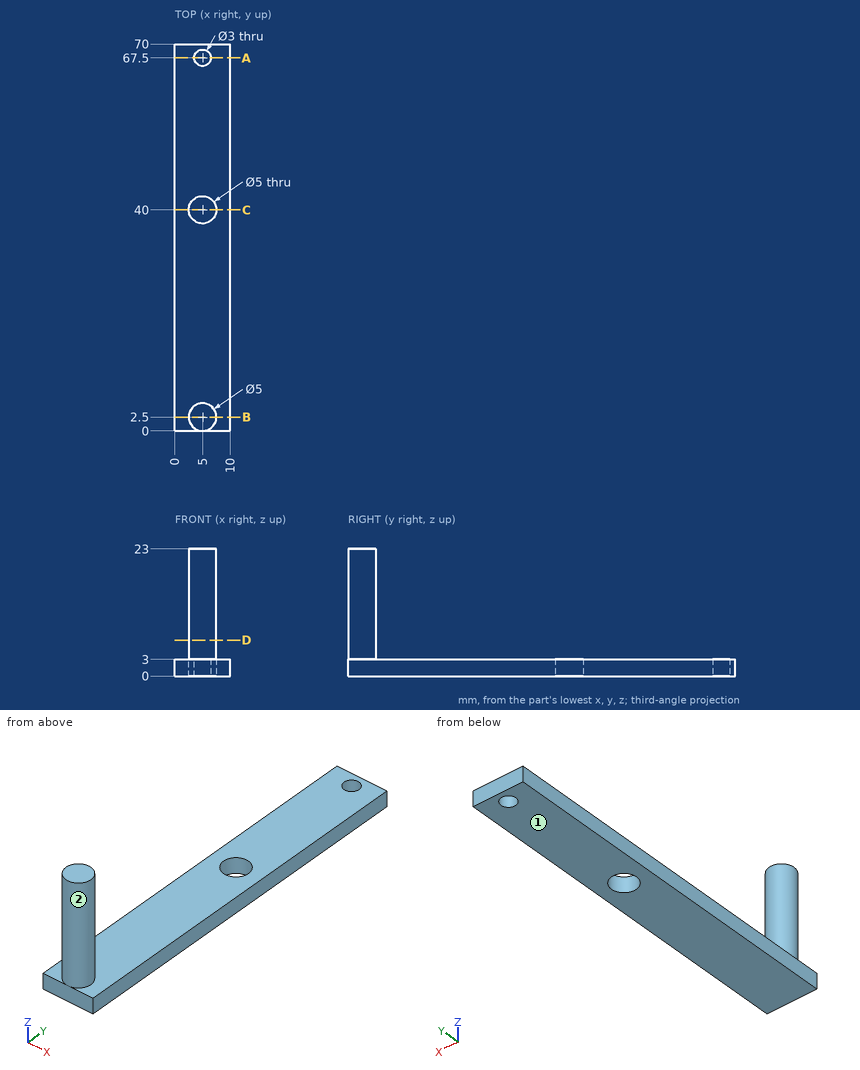
Answer from the drawing. Dimensions are ordinates in mm from the lowest x, y and z of the part. A direction names the side the tool comes from. Coordinates: 2 decimals unless noted, no trailing zeros. Order: outer loops, then holes, each group sorted by start corner. A loop starts at its lowest first (then second) coordinate and runs counter-clockwise, first axis right, second up. Notation, with made-up numbers: M -32.75,25.5 L -26.75,25.5 A33 cw -26.75,60.5 Z; hole C -21.75,15 d11. An arc over 180 degrees is marked long. Put each result on its own line as item: value. Start each with the question number.
Item 1: Section A-A, the plane y = 67.5 is taken. Determine the outline of the cut face in (x, z), plus the area to 3 significant figures.
Item 2: Section D-D, the plane z = 6.5 is taken. Determine the outline of the cut face in (x, y).
Item 3: Consider probe 1 along Y at (x, z) = (5, 1.1); probe 2 along X at (y, z) = (67.5, 1.6); probe 3 along Z at (x, y) = (7.5, 54). Determine where each line is inside the solid, lowest interval first. Write a range as [from, to].
Item 4: For the marked faces 1 and 2, determine the directions among +Z, -Z, +X, -X, +Y, -Y from which every point of the face is accessible in a straight line to the end or side of a thin tool.
Item 5: Given pin 1 Ø2.5 at (x, y) = (5, 67.5) entering from -Z; pin 2 Ø6 at (x, z) = (3.5, 18.5) entering from +Y; pin 3 Ø3 at (x, y) = (3.5, 32.5) entering from +Z, each flat-ended and moving along its own axis, determine where each tip first touches the part or whether it passes through.
Item 6: Section C-C, the plane y = 40 is taken. Determine the outline of the cut face in (x, z), plus the area to 3 significant figures.
Item 7: Section B-B, the plane y = 2.5 is taken. Determine the outline of the cut face in (x, z), plus the area to 3 significant figures.
Computed:
1. outline: M 0,0 L 3.5,0 L 3.5,3 L 0,3 Z; M 6.5,0 L 10,0 L 10,3 L 6.5,3 Z
1. area: 21.0 mm2
2. outline: C 5,2.5 d5
3. probe 1: y = [0, 37.5], [42.5, 66], [69, 70]
3. probe 2: x = [0, 3.5], [6.5, 10]
3. probe 3: z = [0, 3]
4. face 1: -Z, +X, -X, +Y, -Y
4. face 2: +Z
5. pin 1: passes through
5. pin 2: stops at y = 5
5. pin 3: stops at z = 3
6. outline: M 0,0 L 2.5,0 L 2.5,3 L 0,3 Z; M 7.5,0 L 10,0 L 10,3 L 7.5,3 Z
6. area: 15.0 mm2
7. outline: M 0,0 L 10,0 L 10,3 L 7.5,3 L 7.5,23 L 2.5,23 L 2.5,3 L 0,3 Z
7. area: 130 mm2
